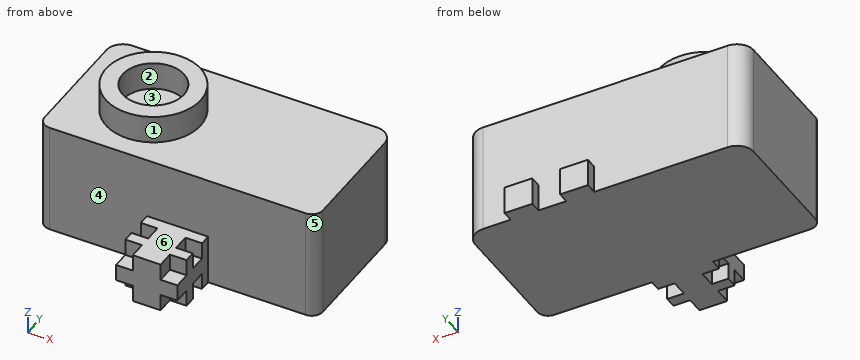
from build123d import *

# Parameters (mm, degrees)
BOSS_EXTRUDE1_DEPTH = 20
SKETCH2_W           = 5
SKETCH2_H           = 2
CUT_EXTRUDE1_DEPTH  = 15
SKETCH3_R           = 8.5
SKETCH3_R_2         = 5.5
BOSS_EXTRUDE2_DEPTH = 5
SKETCH4_W           = 11
SKETCH4_H           = 9
BOSS_EXTRUDE3_DEPTH = 10
SKETCH5_W           = 3
SKETCH5_H           = 3
CUT_EXTRUDE2_DEPTH  = 3
CUT_EXTRUDE3_START  = -8
SKETCH5_2_W         = 3
SKETCH5_2_H         = 3
CUT_EXTRUDE3_DEPTH  = 3


with BuildPart() as part:
    # Sketch1 → Boss-Extrude1 (new body)
    with BuildSketch(Plane.XY):
        with BuildLine():
            Line((-25, 10), (-25, -10))
            ThreePointArc((-25, -10), (-24.414213562, -11.414213562), (-23, -12))
            Line((-23, -12), (23, -12))
            ThreePointArc((23, -12), (24.414213562, -11.414213562), (25, -10))
            Line((25, -10), (25, 10))
            ThreePointArc((25, 10), (24.121320344, 12.121320344), (22, 13))
            Line((22, 13), (17, 13))
            Line((17, 13), (17, 15))
            Line((17, 15), (12, 15))
            Line((12, 15), (12, 13))
            Line((12, 13), (7, 13))
            Line((7, 13), (7, 15))
            Line((7, 15), (2, 15))
            Line((2, 15), (2, 13))
            Line((2, 13), (-22, 13))
            ThreePointArc((-22, 13), (-24.121320344, 12.121320344), (-25, 10))
        make_face()
    extrude(amount=BOSS_EXTRUDE1_DEPTH)

    # Sketch2 → Cut-Extrude1 (cut)
    with BuildSketch(Plane.XY.offset(20)):
        with Locations((4.5, 14)):
            Rectangle(SKETCH2_W, SKETCH2_H)
        with Locations((14.5, 14)):
            Rectangle(SKETCH2_W, SKETCH2_H)
    extrude(amount=-CUT_EXTRUDE1_DEPTH, mode=Mode.SUBTRACT)

    # Sketch3 → Boss-Extrude2 (add)
    with BuildSketch(Plane.XY.offset(20)):
        with Locations((-11, 0)):
            Circle(SKETCH3_R)
        with Locations((-11, 0)):
            Circle(SKETCH3_R_2, mode=Mode.SUBTRACT)
    extrude(amount=BOSS_EXTRUDE2_DEPTH)

    # Sketch4 → Boss-Extrude3 (add)
    with BuildSketch(Plane.XZ.offset(12)):
        with Locations((0, 4.5)):
            Rectangle(SKETCH4_W, SKETCH4_H)
    extrude(amount=BOSS_EXTRUDE3_DEPTH)

    # Sketch5 → Cut-Extrude2 (cut)
    with BuildSketch(Plane(origin=(5.5, 0, 0), x_dir=(0, 0, -1), z_dir=(1, 0, 0))):
        with Locations((-7.5, -20.5)):
            Rectangle(SKETCH5_W, SKETCH5_H)
        with Locations((-1.5, -20.5)):
            Rectangle(SKETCH5_W, SKETCH5_H)
        with Locations((-7.5, -15.5)):
            Rectangle(SKETCH5_W, SKETCH5_H)
        with Locations((-1.5, -15.5)):
            Rectangle(SKETCH5_W, SKETCH5_H)
    extrude(amount=-CUT_EXTRUDE2_DEPTH, mode=Mode.SUBTRACT)

    # Sketch5<2> → Cut-Extrude3 (cut)
    with BuildSketch(Plane(origin=(5.5, 0, 0), x_dir=(0, 0, -1), z_dir=(1, 0, 0)).offset(CUT_EXTRUDE3_START)):
        with Locations((-7.5, -20.5)):
            Rectangle(SKETCH5_2_W, SKETCH5_2_H)
        with Locations((-1.5, -20.5)):
            Rectangle(SKETCH5_2_W, SKETCH5_2_H)
        with Locations((-7.5, -15.5)):
            Rectangle(SKETCH5_2_W, SKETCH5_2_H)
        with Locations((-1.5, -15.5)):
            Rectangle(SKETCH5_2_W, SKETCH5_2_H)
    extrude(amount=-CUT_EXTRUDE3_DEPTH, mode=Mode.SUBTRACT)


solid = part.part
For this review, take the finished solid that the model builds, in its own axes (mm). Face numbers are marked on the shaded views. A direction names the side the tool comes from. Give positions to 0.01 mm unless a question says otherwise; leave off trailing zeros. Loops run counter-clockwise (first coordinate to the right, second up) from the corner with the lowest first, then second, coordinate; pieces in that order, holes last.
Item 1: Tool access review of the marked faces 5 and 6: name each direction out of +Z, -Z, +X, -X, +Y, -Y from which nothing blocks a thin tool from reaching the whole face with its end or side.
Item 2: For line 1 along Y through (x, z) = (-11, 21.45); line 2 along Z through (x, y) = (6.5, 0.5); line 3 along Z through (x, y) = (-1, -19), list the stretches that pass through material, from the lowest coordinate up.
Item 3: Take a section at B-B, the plane z = 15. State the section outline as (x, y) points, and give its area (3 significant figures).
Item 4: Draft analysis for pull direction X (two halves, no side actions). For the marked faces 1, 2, 3 and 4, state which applies: +X half, -X half, draft (parallel to the pull), parting line (faces both ways), or undercut.
Item 5: Take a section at A-A, the plane x = -18.5. State the section outline as (y, z) points, and give its area (3 significant figures).
Item 6: Take a section at D-D, the plane z = 20.75. State the section outline as (x, y) points.
Item 7: Insertion check: pin 1 (11 mm diameter, centred on x = 0, y = -18.5, fed in from +Z); pin 2 (0.9 mm diameter, centred on x = -4, z = 1.5, fed in from -Y); pin 3 (3.5 mm diameter, centred on y = -16, z = 1.5, fed in from -X). Each pin has a flat end and moves straight along its axis. Give the tip position at first contact, or say it passes through.
Item 8: Take a section at C-C, the plane y = 0. State the section outline as (x, z) points, and give its area (3 significant figures).
Calculated:
1. face 5: +Z, -Z, +X, -Y
1. face 6: +Z, +X, -X, -Y
2. line 1: y = -8.5 to -5.5, 5.5 to 8.5
2. line 2: z = 0 to 20
2. line 3: z = 0 to 9
3. outline: (-25, -10) arc R2 ccw to (-23, -12) - (23, -12) arc R2 ccw to (25, -10) - (25, 10) arc R3 ccw to (22, 13) - (-22, 13) arc R3 ccw to (-25, 10) - close
3. area: 1,240 mm2
4. face 1: parting line
4. face 2: undercut
4. face 3: undercut
4. face 4: draft
5. outline: (-12, 0) - (13, 0) - (13, 20) - (4, 20) - (4, 25) - (-4, 25) - (-4, 20) - (-12, 20) - close
5. area: 540 mm2
6. outline: circle Ø17 at (-11, 0); hole circle Ø11 at (-11, 0)
7. pin 1: stops at z = 9
7. pin 2: stops at y = -19
7. pin 3: stops at x = -5.5
8. outline: (-25, 0) - (25, 0) - (25, 20) - (-2.5, 20) - (-2.5, 25) - (-5.5, 25) - (-5.5, 20) - (-16.5, 20) - (-16.5, 25) - (-19.5, 25) - (-19.5, 20) - (-25, 20) - close
8. area: 1,030 mm2
